Part model, mm, in its own coordinate system. A direction names the side the tool comes from. Round coordinates to 2 decimals unless told otherwise and drop trailing zeros. Write each loop counter-clockwise with the first axis right and the second up, starting at its lowest first coordinate (ties: lowest second). Pieces come first, ordered by that corner, then holes. Notation, with made-up numbers: (74.25, 85.5) -> (96.25, 85.5) arc R34 cw to (96.25, 117.5) -> close; hole circle Ø1 at (-39, 11.5). An arc over 180 degrees is marked (long way). Return JSON: item names as keys, results as strings. Group by question number.
(1) Saw through at A-A (z = 2.3). List the corners of the cut face in (x, y), plus the area to 3 significant figures.
(2) Saw through at C-C (y = -54). List the corners of the cut face in (x, z), plus the area to 3 significant figures.
(3) Saw through at B-B (x = 27.5). List the corners of the cut face in (y, z).
(4) Mould opens along Y. For faces 1 (the flat face through (25, -3, 2)), 2 (the flat face through (3, -53, 2)), 3 (the flat face through (1, -18, 2)) say: +Y half, -Y half, draft (parallel to the pull), parting line (faces both ways), or undercut.
(5) Tool access for faces 4 (the flat face through (30, -2, 2)), 5 (the flat face through (1, -38, 2)), 6 (the flat face through (55, 0, 1)), 7 (the flat face through (39, -29, 0)), 8 (the flat face through (10, -2, 2)): list every direction of +Z, -Z, +X, -X, +Y, -Y with a clear straight run to the whole face (end or side of a thin tool).
(6) Drill centre lines: L1, parallel to Y at x = 27, z = 2.4; L2, parallel to X at y = -13, z = 1.25. Where is each one in solid material? Low to high. Write a range as from..to.
(7) Drop flat-ended pins along their axis: pin 1 Ø1.5 at (x, z) = (3, 1.5) entering from +Y; pin 2 Ø0.9 at (y, z) = (-31, 2) entering from -X; pin 3 Ø1.5 at (x, z) = (36.5, 1) entering from +Y; pin 4 Ø1.5 at (x, z) = (1, 1) entering from -Y. Give the stop position or say it passes through.
from build123d import *

# Parameters (mm, degrees)
ESQUISSE1_W                = 80
ESQUISSE1_H                = 58
BOSS_EXTRU_1_DEPTH         = 3
ESQUISSE2_W                = 10
ESQUISSE2_H                = 3
ENL_V_MAT_EXTRU_1_DEPTH    = 4
R_P_TITION_LIN_AIRE1_COUNT = 4
R_P_TITION_LIN_AIRE1_PITCH = 20
ESQUISSE3_W                = 3
ESQUISSE3_H                = 10
ENL_V_MAT_EXTRU_2_DEPTH    = 4
R_P_TITION_LIN_AIRE2_COUNT = 3
R_P_TITION_LIN_AIRE2_PITCH = 20


with BuildPart() as part:
    # Esquisse1 → Boss.-Extru.1 (new body)
    with BuildSketch(Plane.XY):
        with Locations((40, -29)):
            Rectangle(ESQUISSE1_W, ESQUISSE1_H)
    extrude(amount=BOSS_EXTRU_1_DEPTH)

    # Esquisse2 → Enlèv. mat.-Extru.1 (cut, through all)
    with BuildSketch(Plane.XY.offset(3)):
        with Locations((5, -1.5)):
            Rectangle(ESQUISSE2_W, ESQUISSE2_H)
    enl_v_mat_extru_1 = extrude(amount=-ENL_V_MAT_EXTRU_1_DEPTH, mode=Mode.SUBTRACT)

    # Répétition linéaire1: Enlèv. mat.-Extru.1 ×4
    with Locations(*[(i * R_P_TITION_LIN_AIRE1_PITCH, 0, 0) for i in range(1, R_P_TITION_LIN_AIRE1_COUNT)]):
        add(enl_v_mat_extru_1, mode=Mode.SUBTRACT)

    # Esquisse3 → Enlèv. mat.-Extru.2 (cut, through all)
    with BuildSketch(Plane.XY.offset(3)):
        with Locations((1.5, -53)):
            Rectangle(ESQUISSE3_W, ESQUISSE3_H)
    enl_v_mat_extru_2 = extrude(amount=-ENL_V_MAT_EXTRU_2_DEPTH, mode=Mode.SUBTRACT)

    # Répétition linéaire2: Enlèv. mat.-Extru.2 ×3
    with Locations(*[(0, i * R_P_TITION_LIN_AIRE2_PITCH, 0) for i in range(1, R_P_TITION_LIN_AIRE2_COUNT)]):
        add(enl_v_mat_extru_2, mode=Mode.SUBTRACT)


solid = part.part
Computed values:
{
 "1": {"outline": "(0, -48) -> (3, -48) -> (3, -58) -> (80, -58) -> (80, 0) -> (70, 0) -> (70, -3) -> (60, -3) -> (60, 0) -> (50, 0) -> (50, -3) -> (40, -3) -> (40, 0) -> (30, 0) -> (30, -3) -> (20, -3) -> (20, 0) -> (10, 0) -> (10, -3) -> (0, -3) -> (0, -8) -> (3, -8) -> (3, -18) -> (0, -18) -> (0, -28) -> (3, -28) -> (3, -38) -> (0, -38) -> close", "area": "4,430 mm2"},
 "2": {"outline": "(3, 0) -> (80, 0) -> (80, 3) -> (3, 3) -> close", "area": "231 mm2"},
 "3": {"outline": "(-58, 0) -> (-3, 0) -> (-3, 3) -> (-58, 3) -> close"},
 "4": {"face 1": "+Y half", "face 2": "draft", "face 3": "undercut"},
 "5": {"face 4": "+Z, -Z, +Y", "face 5": "+Z, -Z, -X", "face 6": "+Z, -Z, +X, -X, +Y", "face 7": "-Z, +X, -X, +Y, -Y", "face 8": "+Z, -Z, -X, +Y"},
 "6": {"L1": "-58..-3", "L2": "3..80"},
 "7": {"pin 1": "y = -3", "pin 2": "x = 3", "pin 3": "y = 0", "pin 4": "y = -48"}
}
